from build123d import *

# Parameters (mm, degrees)
F0_R     = 1.5
F1_DEPTH = 10


with BuildPart() as f1:
    # F0 (on Front) → F1 (new body, symmetric)
    with BuildSketch(Plane.XZ):
        Polygon((79.5, 0), (0, 0), (0, -4.123699), (10, -4.123699), (10, -7.245275), (72.830607, -18.324006), align=None)
        with Locations((40, -6)):
            Circle(F0_R, mode=Mode.SUBTRACT)
        with Locations((60, -6)):
            Circle(F0_R, mode=Mode.SUBTRACT)
    extrude(amount=F1_DEPTH, both=True)


solid = f1.part
Verification items for the finished model (mm, model axes). A direction names the side the tool comes from. Round coordinates to 2 decimals unless told otherwise and drop trailing zeros. Write each loop counter-clockwise with the first axis right and the second up, starting at its lowest first coordinate (ties: lowest second). Pieces come first, ordered by that corner, then holes.
(1) Section check A-A (x = 40). Enter the section's corners in (y, z).
Returned:
outline: (-10, -12.54) - (10, -12.54) - (10, -7.5) - (-10, -7.5) - close; (-10, -4.5) - (10, -4.5) - (10, 0) - (-10, 0) - close
(2) Access from +Z, -Z, +X, -X, +Y, -Y to the whole of each face (thin tool, end or side, straight path). Record for faces 1 (the flat face through (76.12, -0.14, -9.29)), 2 (the flat face through (5, 0, -4.124)).
Returned:
face 1: -Z, +X, +Y, -Y
face 2: -Z, -X, +Y, -Y
(3) Depth check by flat-ended pin: pin 1 Ø1.5 at (y, z) = (7, -2) entering from +X; pin 2 Ø2.5 at (y, z) = (4, -5.5) entering from -X; pin 3 Ø5 at (x, y) = (7, 2.5) entering from -Z. Enter the tip coordinate at first touch or a pass-through.
Returned:
pin 1: stops at x = 79.05
pin 2: stops at x = 10
pin 3: stops at z = -4.12
(4) Section check B-B (z = -6). Enter the section's corners in (x, y), plus the area to 3 significant figures.
Returned:
outline: (10, -10) - (38.5, -10) - (38.5, 10) - (10, 10) - close; (41.5, -10) - (58.5, -10) - (58.5, 10) - (41.5, 10) - close; (61.5, -10) - (77.32, -10) - (77.32, 10) - (61.5, 10) - close
area: 1,230 mm2
(5) Material ranges on line 1 (Z direction, x = 5.5, y = 3.5); line 2 (Z direction, x = 40, y = -2.75); line 3 (Z direction, x = 60, y = 2), recorded low to high.
Returned:
line 1: z = -4.12 to 0
line 2: z = -12.54 to -7.5, -4.5 to 0
line 3: z = -16.06 to -7.5, -4.5 to 0
(6) Section check D-D (x = 6). Enter the section's corners in (y, z).
Returned:
outline: (-10, -4.12) - (10, -4.12) - (10, 0) - (-10, 0) - close
(7) Mould release check, pull along X, two halves, no side actions. Record for faces 3 (the flat face through (10, 0, -6)), 4 (the cylindrical face through (61.43, 0.14, -5.55)), 5 (the flat face through (48, -10, -7)): pulls with the +X half, pulls with the -X half, needs draft (parallel to the pull), parting line crosses it, or undercut.
Returned:
face 3: pulls with the -X half
face 4: undercut
face 5: needs draft
(8) Section check C-C (y = -4.25). Enter the section's corners in (x, z), plus the area to 3 significant figures.
Returned:
outline: (0, -4.12) - (10, -4.12) - (10, -7.25) - (72.83, -18.32) - (79.5, 0) - (0, 0) - close; hole circle Ø3 at (40, -6); hole circle Ø3 at (60, -6)
area: 891 mm2
